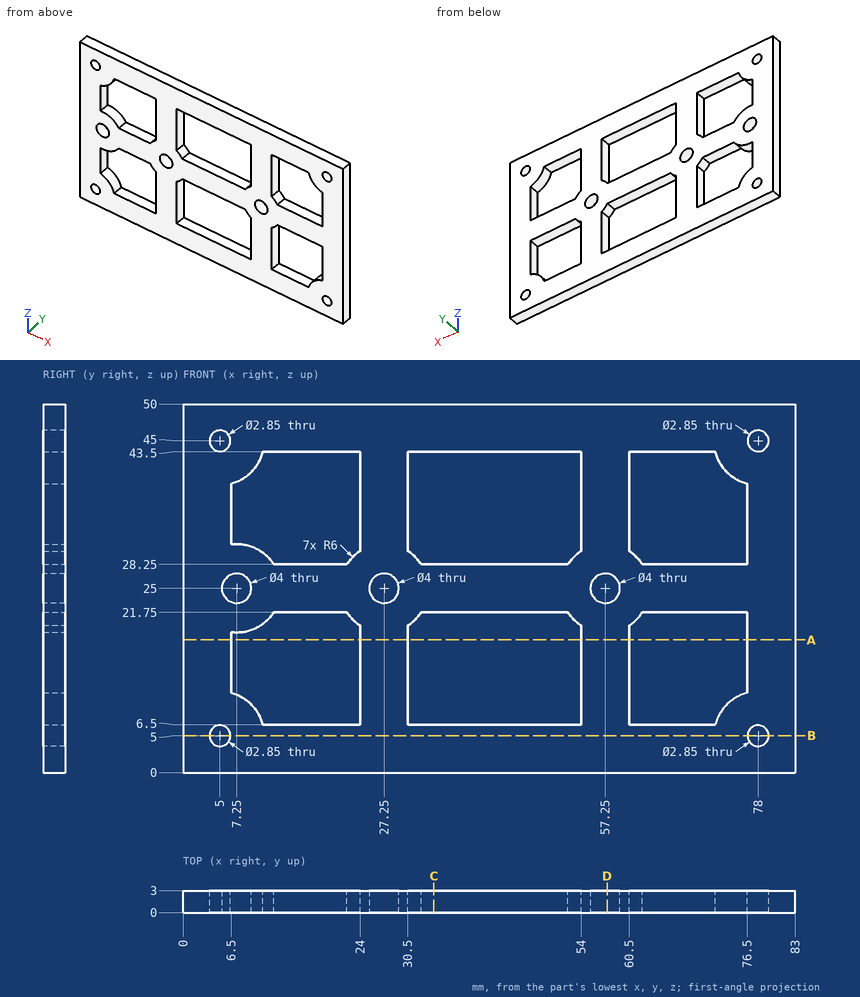
Here's the drawing with two shaded views (mm, measured from the low corner). I have some questions. Round coordinates to 2 decimals unless told otherwise and drop trailing zeros. Write each loop counter-clockwise with the first axis right and the second up, starting at its lowest first coordinate (ties: lowest second). Pieces come first, ordered by that corner, then holes. Notation, with made-up numbers: M 76.25,36.5 L 103.25,36.5 A20 cw 103.25,63.5 Z; hole C -31,73.5 d6. An arc over 180 degrees is marked long. Answer in a Markdown table with one row per item. Add a question column.
Q1. If I drill on line 1 (Z direction, x = 70.5, y = 0.2); line 2 (X direction, y = 1.8, z = 45) (3 decimals); line 3 (X direction, y = 2.55, z = 35.5), over which ranges is the centre line in solid material (lowest first)? Write a range as from..to.
Q2. Imagine slicing it at D-D (x = 57.5). Please give me the cut outline in (y, z), then the cut area to 3 significant figures.
Q3. Imagine slicing it at C-C (x = 34). Please give me the cut outline in (y, z).
Q4. Imagine slicing it at B-B (z = 5). Please give me the cut outline in (x, y) (3 decimals).
Q5. Imagine slicing it at A-A (z = 18). Please give me the cut outline in (x, y), then the cut area to 3 significant figures.
Q6. Will this pin go through, and if not, where does the flat tip stop? pin 1 Ø4.5 at (x, z) = (57.25, 25) entering from -Y.
Values:
| question | item | result |
|---|---|---|
| 1 | line 1 | 0..6.5, 21.75..28.25, 43.5..50 |
| 1 | line 2 | 0..3.575, 6.425..76.575, 79.425..83 |
| 1 | line 3 | 0..6.5, 24..30.5, 54..60.5, 76.5..83 |
| 2 | outline | M 0,0 L 3,0 L 3,23.02 L 0,23.02 Z; M 0,26.98 L 3,26.98 L 3,50 L 0,50 Z |
| 2 | area | 138 mm^2 |
| 3 | outline | M 0,0 L 3,0 L 3,6.5 L 0,6.5 Z; M 0,21.75 L 3,21.75 L 3,28.25 L 0,28.25 Z; M 0,43.5 L 3,43.5 L 3,50 L 0,50 Z |
| 4 | outline | M 0,0 L 3.575,0 L 3.575,3 L 0,3 Z; M 6.425,0 L 76.575,0 L 76.575,3 L 6.425,3 Z; M 79.425,0 L 83,0 L 83,3 L 79.425,3 Z |
| 5 | outline | M 0,0 L 6.5,0 L 6.5,3 L 0,3 Z; M 24,0 L 30.5,0 L 30.5,3 L 24,3 Z; M 54,0 L 60.5,0 L 60.5,3 L 54,3 Z; M 76.5,0 L 83,0 L 83,3 L 76.5,3 Z |
| 5 | area | 78.0 mm^2 |
| 6 | pin 1 | y = 0 |
